Part model, mm, in its own coordinate system. A direction names the side the tool comes from. Round coordinates to 2 decimals unless told otherwise and drop trailing zeros. Write each loop counter-clockwise with the first axis right and the second up, starting at its lowest first coordinate (ties: lowest second). Pieces come first, ordered by that corner, then holes. Notation, with made-up numbers: (-36, -3.5) -> (17, -3.5) arc R16 ccw to (17, 6.5) -> close; hole circle Ø2 at (30.25, 39.5). An arc over 180 degrees is marked (long way). Return JSON: item names as keys, results as strings. Group by question number.
Autodesk Fusion 360 part; units mm, degrees
sketch "Sketch1" plane through (0, 0, 0) normal (0, 1, 0) x (1, 0, 0)
  circle A0 centre (0, 0) radius 1.45
  circle A1 centre (0, 0) radius 15
  dimension "d1" = 2.9
  dimension "d2" = 30
extrude "Extrude1" add sketch "Sketch1" along normal blind 12
extrude "Extrude2" add sketch "Sketch1" along normal blind 4 contours A0
fillet "Fillet1" radius 1 1 edges at (-1.3519, 12, -0.5243)
sketch "Sketch2" plane through (0, 12, 0) normal (0, 1, 0) x (-1, 0, 0)
  circle A0 centre (0, 0) radius 15
  circle A1 centre (0, 0) radius 2.45
  circle A2 centre (0, 0) radius 7.5
  dimension "d8" = 15
extrude "Extrude3" cut sketch "Sketch2" against normal blind 4 contours A0
fillet "Fillet2" radius 3 1 edges at (-13.9849, 0, 5.4242)
fillet "Fillet3" radius 2 1 edges at (-13.9849, 8, -5.4242)
Item 1: Cut at A-A (z = 0). Write the cut outline in (x, y), then the cut area to 3 significant figures.
Item 2: Cut at C-C (y = 6.75). Write the cut outline in (x, z).
Item 3: Which spindle directions (+Z, -Z, +X, -X, +Y, -Y) get a long thin tool onto all of the face, cutting with end or side? Do faces 5 (the face through (0, 0, 0)), 6 (the face through (7.493, 10.028, 0.33)). Say none if no direction does.
Item 4: Two-plate mould, pull along X, no slides. Class faces 1 (the face through (-1.45, 7.45, 0.06)), 2 (the face through (-14.985, 4.479, 0.66)), 3 (the face through (-2, 12, -2)), 4 (the face through (0, 4, 0)): released by +X, released by -X, zero draft, split by the parting line, or undercut.
Item 5: Flat gauge pins, fed straight in: P1, Ø2, axis at x = -7, y = 7, coming from the -Z side; P2, Ø1, axis at y = 4.5, z = -1, coming from the -X side; P3, Ø1.4, axis at x = 0, z = -0.5, coming from the +Y side. Where does each tip first touch, or does it go through?
Item 6: Cut at B-B (x = 0). Write the cut outline in (y, z), then the cut area to 3 significant figures.
Item 7: Wall check: L1, parallel to Y at x = -7.75, z = 5.5; L2, parallel to Z at x = 0, y = 9; L3, parallel to X at y = 5.5, z = 0. Give the ranges that are in metal, low to high.
Checks:
{
 "1": {"outline": "(-15, 3) arc R3 ccw to (-12, 0) -> (12, 0) arc R3 ccw to (15, 3) -> (15, 6) arc R2 ccw to (13, 8) -> (7.5, 8) -> (7.5, 12) -> (2.45, 12) arc R1 ccw to (1.45, 11) -> (1.45, 4) -> (-1.45, 4) -> (-1.45, 11) arc R1 ccw to (-2.45, 12) -> (-7.5, 12) -> (-7.5, 8) -> (-13, 8) arc R2 ccw to (-15, 6) -> close", "area": "271 mm2"},
 "2": {"outline": "circle Ø29.71 at (0, 0); hole circle Ø2.9 at (0, 0)"},
 "3": {"face 5": "+Z, -Z, +X, -X, -Y", "face 6": "+Y"},
 "4": {"face 1": "undercut", "face 2": "split by the parting line", "face 3": "zero draft", "face 4": "undercut"},
 "5": {"P1": "stops at z = -13.62", "P2": "stops at x = -14.99", "P3": "stops at y = 4"},
 "6": {"outline": "(0, -12) arc R3 ccw to (3, -15) -> (6, -15) arc R2 ccw to (8, -13) -> (8, -7.5) -> (12, -7.5) -> (12, -2.45) arc R1 ccw to (11, -1.45) -> (4, -1.45) -> (4, 1.45) -> (11, 1.45) arc R1 ccw to (12, 2.45) -> (12, 7.5) -> (8, 7.5) -> (8, 13) arc R2 ccw to (6, 15) -> (3, 15) arc R3 ccw to (0, 12) -> close", "area": "271 mm2"},
 "7": {"L1": "y = 0 to 8", "L2": "z = -7.5 to -1.45, 1.45 to 7.5", "L3": "x = -15 to -1.45, 1.45 to 15"}
}
